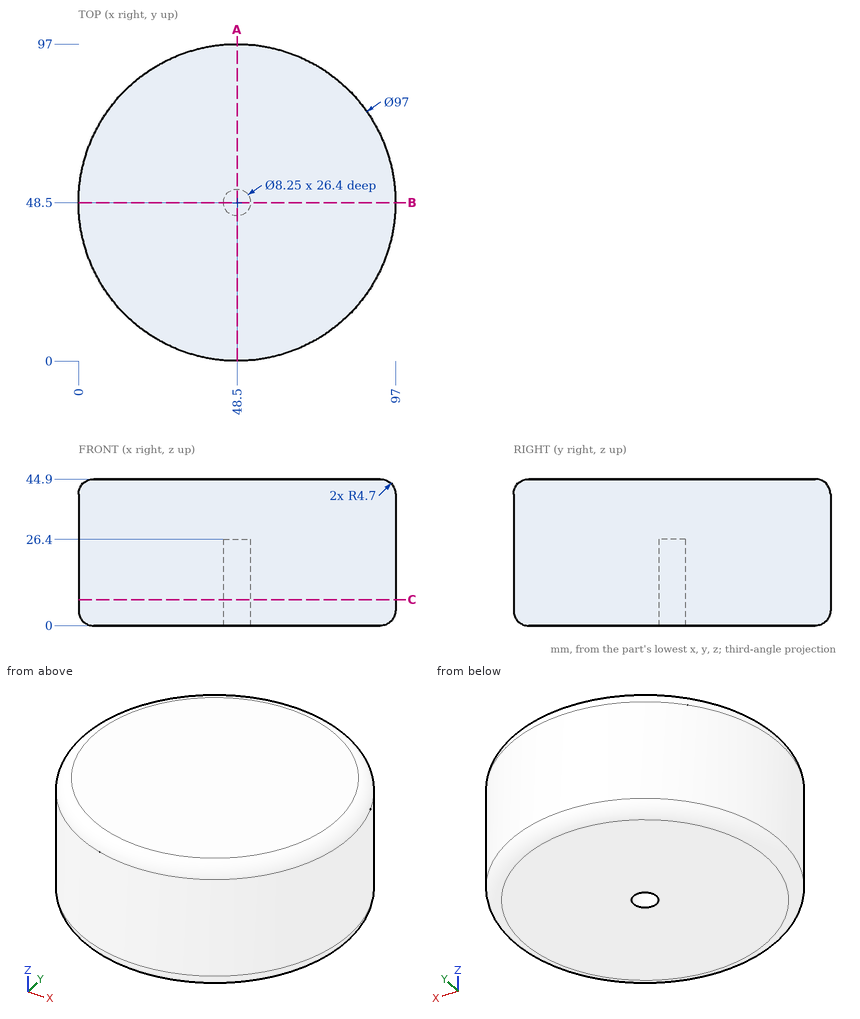
Source: three-view drawing plus pictorial views. Frame: mm from the lowest corner of the part. Give positions to 0.01 mm unless a question says otherwise; leave off trailing zeros. Order: outer loops, then holes, each group sorted by start corner. A loop starts at its lowest first (then second) coordinate and runs counter-clockwise, first axis right, second up. Notation, with made-up numbers: M 73.5,-18 L 105.5,-18 A22 cw 105.5,-4 Z; hole C -32,62 d10. An arc over 180 degrees is marked long. One line per question, with ' | ' between items. Start each with the question number.
1. First-contact query: pin 1 Ø3 at (y, z) = (66.5, 7.5) entering from +X; pin 2 Ø6 at (x, z) = (45.5, 24) entering from +Y; pin 3 Ø1 at (y, z) = (61.5, 19) entering from +X. Flat tips, straight axial feed; report the tip coordinate or a pass-through.
2. Material intervals for probe 1 along Y at (x, z) = (48.5, 12.25) (3 decimals); probe 2 along X at (y, z) = (48, 40.5); probe 3 along X at (y, z) = (46.5, 15.5), sorted ascending. Write a range as [from, to].
3. Section query A-A (x = 48.5). Return the cut outline in (y, z) (3 decimals).
4. Section query C-C (z = 8). Return the cut outline in (x, y) (3 decimals).
Here are the results:
1) pin 1: x = 94.11 | pin 2: y = 97 | pin 3: x = 95.36
2) probe 1: [0, 44.375], [52.625, 97] | probe 2: [0.01, 96.99] | probe 3: [0.04, 44.89], [52.11, 96.96]
3) outline: M 0,4.7 A4.7 ccw 4.7,0 L 44.375,0 L 44.375,26.4 L 52.625,26.4 L 52.625,0 L 92.3,0 A4.7 ccw 97,4.7 L 97,40.2 A4.7 ccw 92.3,44.9 L 4.7,44.9 A4.7 ccw 0,40.2 Z
4) outline: C 48.5,48.5 d97; hole C 48.5,48.5 d8.25
